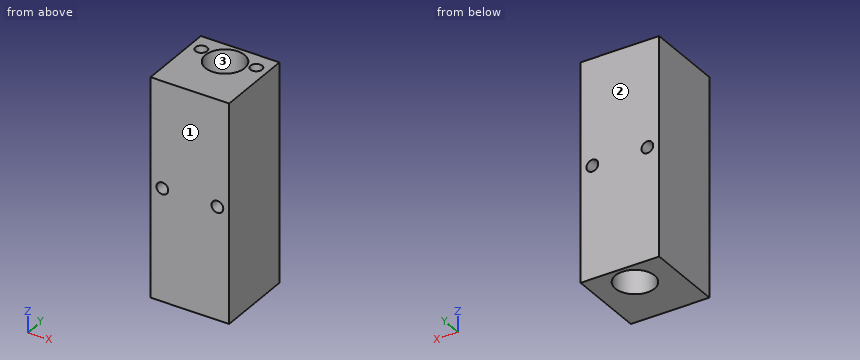
Autodesk Inventor part; units mm, degrees
ref_plane "YZ Plane" through (0, 0, 0) normal (1, 0, 0) x (0, 1, 0)
ref_plane "XZ Plane" through (0, 0, 0) normal (0, 1, 0) x (-1, 0, 0)
ref_plane "XY Plane" through (0, 0, 0) normal (0, 0, 1) x (1, 0, 0)
sketch "Sketch1" plane through (0, 0, 0) normal (0, 0, 1) x (1, 0, 0)
  line L0 (0, 0) -> (20, 0)
  line L1 (20, 0) -> (20, 20)
  line L2 (20, 20) -> (0, 20)
  line L3 (0, 20) -> (0, 0)
  dimension "d0" = 20
  dimension "d1" = 20
extrude "Extrusion1" add sketch "Sketch1" along normal blind 55.5
sketch "Sketch2" plane through (0, 0, 0) normal (0, -1, 0) x (1, 0, 0)
  circle A0 centre (17, 28.5) radius 1.5
  circle A1 centre (3, 28.5) radius 1.5
  line L0 (0, 0) -> (20, 0)
  dimension "d4" = 14
  dimension "d5" = 3
  dimension "d6" = 28.5
  dimension "d7" = 3
  dimension "d8" = 3
extrude "Extrusion2" cut sketch "Sketch2" against normal through all
sketch "Sketch3" plane through (0, 0, 55.5) normal (0, 0, 1) x (1, 0, 0)
  circle A0 centre (17, 15.5) radius 1.5
  circle A1 centre (3, 15.5) radius 1.5
  line L0 (0, 20) -> (0, 0)
  line L1 (20, 0) -> (20, 20)
  line L2 (20, 20) -> (0, 20)
  dimension "d11" = 3
  dimension "d12" = 3
  dimension "d13" = 14
  dimension "d14" = 3
  dimension "d15" = 3
  dimension "d22" = 4.5
extrude "Extrusion3" cut sketch "Sketch3" against normal blind 10
sketch "Sketch4" plane through (0, 0, 55.5) normal (0, 0, 1) x (1, 0, 0)
  circle A0 centre (10, 14) radius 5
  line L0 (20, 20) -> (0, 20)
  point P0 (0, 0)
  point P1 (10, 20)
  dimension "d18" = 6
  dimension "d19" = 10
extrude "Extrusion4" cut sketch "Sketch4" against normal through all
sketch "Sketch5" plane through (0, 20, 0) normal (0, 1, 0) x (1, 0, 0)
  point P0 (0, 0)
properties part number "BLOQUE_PRESION"
Here's how the part is built. I have some questions about the finished solid (model axes, mm). Face numbers are marked on the shaded views. Round coordinates to 2 decimals unless told otherwise and drop trailing zeros. Write each loop counter-clockwise with the first axis right and the second up, starting at its lowest first coordinate (ties: lowest second). Pieces come first, ordered by that corner, then holes.
Q1. If we section it at A-A on y = 11: Write out the boundary of the cut face in (x, z).
Q2. If we section it at C-C on x = 10: Write out the boundary of the cut face in (y, z).
Q3. Will these pins go through, and if not, where does the flat tip stop? P1, Ø4, axis at x = 15.5, y = 5, coming from the -Z side; P2, Ø0.9, axis at x = 17, y = 15, coming from the +Z side.
Q4. If we mould it in two halves opening along Y, with no side actions, what happens to the marked faces 1, 2 and 3? For each: +Y half, -Y half, draft (parallel to the pull), parting line (faces both ways), or undercut.
Q5. If we section it at B-B on x = 3: Write out the boundary of the cut face in (y, z), plus the area to 3 significant figures.
Q6. Please list where these lines run through material, in increasing order: probe 1 along Y at (x, z) = (3, 48.5); probe 2 along Z at (x, y) = (17, 14.5); probe 3 along Y at (x, z) = (10, 33).
Q7. If we section it at D-D on z = 4: Write out the boundary of the cut face in (x, y), plus the area to 3 significant figures.
Answer below:
1. outline: (0, 0) - (6, 0) - (6, 55.5) - (0, 55.5) - close; (14, 0) - (20, 0) - (20, 55.5) - (14, 55.5) - close; hole circle Ø3 at (3, 28.5); hole circle Ø3 at (17, 28.5)
2. outline: (0, 0) - (9, 0) - (9, 55.5) - (0, 55.5) - close; (19, 0) - (20, 0) - (20, 55.5) - (19, 55.5) - close
3. P1: stops at z = 0
3. P2: stops at z = 45.5
4. face 1: -Y half
4. face 2: +Y half
4. face 3: undercut
5. outline: (0, 0) - (20, 0) - (20, 27) - (0, 27) - close; (0, 30) - (20, 30) - (20, 55.5) - (17, 55.5) - (17, 45.5) - (14, 45.5) - (14, 55.5) - (0, 55.5) - close
5. area: 1,020 mm2
6. probe 1: y = 0 to 14, 17 to 20
6. probe 2: z = 0 to 27, 30 to 45.5
6. probe 3: y = 0 to 9, 19 to 20
7. outline: (0, 0) - (20, 0) - (20, 20) - (0, 20) - close; hole circle Ø10 at (10, 14)
7. area: 321 mm2
